```python
from build123d import *

# Parameters (mm, degrees)
F1_DEPTH = 15.24
F2_DEPTH = 12.7
F3_DEPTH = 10.16


with BuildPart() as f1:
    # F0 (on Top) → F1 (new body)
    with BuildSketch(Plane.XY):
        with BuildLine():
            Line((-35.3495, 60.131524), (-40.133959, 60.131524))
            Line((-40.133959, 60.131524), (-40.133959, 43.769562))
            ThreePointArc((-40.133959, 43.769562), (-39.905763, 42.381693), (-39.245203, 41.139955))
            Line((-39.245203, 41.139955), (-26.097199, 34.712043))
            Line((-26.097199, 34.712043), (-26.097199, 60.034128))
            Line((-26.097199, 60.034128), (-30.674654, 60.034128))
            Line((-30.674654, 60.034128), (-30.674654, 42.308667))
            Line((-30.674654, 42.308667), (-30.674654, 42.125131))
            Line((-30.674654, 42.125131), (-34.736989, 43.975933))
            ThreePointArc((-34.736989, 43.975933), (-35.180866, 44.310949), (-35.3495, 44.840879))
            Line((-35.3495, 44.840879), (-35.3495, 60.131524))
        make_face()
        with BuildLine():
            Line((-11.580281, 51.967774), (-6.953094, 49.838448))
            Line((-6.953094, 49.838448), (-6.830248, 58.170216))
            ThreePointArc((-6.830248, 58.170216), (-7.547014, 59.653243), (-9.164316, 59.965426))
            Line((-9.164316, 59.965426), (-19.565252, 59.965426))
            ThreePointArc((-19.565252, 59.965426), (-20.778535, 59.428841), (-21.197871, 58.170216))
            Line((-21.197871, 58.170216), (-21.197871, 47.978059))
            ThreePointArc((-21.197871, 47.978059), (-20.754073, 46.476274), (-19.565252, 45.456952))
            Line((-19.565252, 45.456952), (-11.785025, 41.853478))
            Line((-11.785025, 41.853478), (-11.785025, 35.219812))
            Line((-11.785025, 35.219812), (-14.241938, 34.277995))
            Line((-14.241938, 34.277995), (-16.371263, 35.219812))
            Line((-16.371263, 35.219812), (-16.371263, 39.150875))
            Line((-16.371263, 39.150875), (-21.203195, 41.362097))
            Line((-21.203195, 41.362097), (-21.203195, 34.277995))
            ThreePointArc((-21.203195, 34.277995), (-20.840997, 32.929487), (-19.85189, 31.943927))
            Line((-19.85189, 31.943927), (-13.914351, 29.282272))
            Line((-13.914351, 29.282272), (-8.672934, 31.698236))
            ThreePointArc((-8.672934, 31.698236), (-7.409398, 32.743692), (-6.830248, 34.277995))
            Line((-6.830248, 34.277995), (-6.830248, 43.409521))
            ThreePointArc((-6.830248, 43.409521), (-7.490944, 45.226204), (-9.164316, 46.194026))
            Line((-9.164316, 46.194026), (-16.207468, 49.388015))
            Line((-16.207468, 49.388015), (-16.207468, 55.325555))
            Line((-16.207468, 55.325555), (-11.580281, 55.325555))
            Line((-11.580281, 55.325555), (-11.580281, 51.967774))
        make_face()
        with BuildLine():
            Line((-2.144403, 34.621232), (2.7823, 36.786695))
            Line((2.7823, 36.786695), (2.7823, 41.127243))
            ThreePointArc((2.7823, 41.127243), (3.032611, 41.95286), (3.683167, 42.519495))
            Line((3.683167, 42.519495), (7.368538, 44.239336))
            Line((7.368538, 44.239336), (7.368538, 39.161714))
            Line((7.368538, 39.161714), (10.685371, 40.553966))
            ThreePointArc((10.685371, 40.553966), (11.819683, 41.556771), (12.241417, 43.010876))
            Line((12.241417, 43.010876), (12.241417, 59.792126))
            Line((12.241417, 59.792126), (-0.319427, 59.792126))
            ThreePointArc((-0.319427, 59.792126), (-1.598421, 59.370402), (-2.144403, 58.139313))
            Line((-2.144403, 58.139313), (-2.144403, 34.621232))
        make_face()
        Polygon((2.7823, 47.515221), (2.7823, 55.500185), (7.368538, 55.377342), (7.368538, 49.521698), align=None, mode=Mode.SUBTRACT)
    extrude(amount=F1_DEPTH)


with BuildPart() as f2:
    # F0 (on Top) → F2 (new body)
    with BuildSketch(Plane.XY):
        with BuildLine():
            Line((-36.221196, 34.301637), (-40.116899, 36.103401))
            Line((-40.116899, 36.103401), (-40.26299, 9.51521))
            ThreePointArc((-40.26299, 9.51521), (-38.829457, 4.505833), (-34.924753, 1.055882))
            ThreePointArc((-34.924753, 1.055882), (-35.890099, 3.120786), (-36.221196, 5.376023))
            Line((-36.221196, 5.376023), (-36.221196, 34.301637))
        make_face()
        Polygon((-28.137608, 30.40593), (-32.228097, 32.353785), (-32.053457, -1.11851), (-28.137608, -3.845503), align=None)
        Polygon((-20.025467, 26.800887), (-24.018567, 28.700044), (-24.067261, -6.799573), (-19.834662, -9.769816), align=None)
        Polygon((-14.174307, 24.187266), (-15.983673, 25.047818), (-16.051294, -12.73049), (-13.916418, -14.146952), (-11.990574, -12.73049), (-11.990574, 24.950425), align=None)
        Polygon((-3.661716, 28.700044), (-7.946991, 26.800887), (-7.946991, -9.852093), (-3.476346, -6.828905), align=None)
        Polygon((3.93491, 32.353785), (-0.058187, 30.371067), (-0.058187, -4.008536), (4.109884, -1.182727), align=None)
        with BuildLine():
            Line((12.117932, 36.103401), (7.830616, 33.974593))
            Line((7.830616, 33.974593), (7.984579, 4.465428))
            ThreePointArc((7.984579, 4.465428), (7.646931, 2.635085), (6.661903, 1.055882))
            ThreePointArc((6.661903, 1.055882), (10.736967, 4.274239), (12.258095, 9.23913))
            Line((12.258095, 9.23913), (12.117932, 36.103401))
        make_face()
    extrude(amount=F2_DEPTH)


with BuildPart() as f3:
    # F0 (on Top) → F3 (new body)
    with BuildSketch(Plane.XY):
        with BuildLine():
            Line((17.619875, 65.742654), (-45.880125, 65.742654))
            Line((-45.880125, 65.742654), (-45.880125, 10.423636))
            ThreePointArc((-45.880125, 10.423636), (-44.380848, 3.249228), (-40.133959, -2.724371))
            Line((-40.133959, -2.724371), (-13.956032, -21.107036))
            Line((-13.956032, -21.107036), (13.139814, -1.26348))
            ThreePointArc((13.139814, -1.26348), (16.461486, 4.165449), (17.619875, 10.423636))
            Line((17.619875, 10.423636), (17.619875, 65.742654))
        make_face()
        Polygon((-32.053457, -1.11851), (-32.228097, 32.353785), (-28.137608, 30.40593), (-28.137608, -3.845503), align=None, mode=Mode.SUBTRACT)
        with BuildLine():
            Line((-40.26299, 9.51521), (-40.116899, 36.103401))
            Line((-40.116899, 36.103401), (-36.221196, 34.301637))
            Line((-36.221196, 34.301637), (-36.221196, 5.376023))
            ThreePointArc((-36.221196, 5.376023), (-35.890099, 3.120786), (-34.924753, 1.055882))
            ThreePointArc((-34.924753, 1.055882), (-38.829457, 4.505833), (-40.26299, 9.51521))
        make_face(mode=Mode.SUBTRACT)
        Polygon((-24.067261, -6.799573), (-24.018567, 28.700044), (-20.025467, 26.800887), (-19.834662, -9.769816), align=None, mode=Mode.SUBTRACT)
        Polygon((-16.051294, -12.73049), (-15.983673, 25.047818), (-14.174307, 24.187266), (-11.990574, 24.950425), (-11.990574, -12.73049), (-13.916418, -14.146952), align=None, mode=Mode.SUBTRACT)
        Polygon((-7.946991, -9.852093), (-7.946991, 26.800887), (-3.661716, 28.700044), (-3.476346, -6.828905), align=None, mode=Mode.SUBTRACT)
        Polygon((-0.058187, -4.008536), (-0.058187, 30.371067), (3.93491, 32.353785), (4.109884, -1.182727), align=None, mode=Mode.SUBTRACT)
        with BuildLine():
            Line((7.984579, 4.465428), (7.830616, 33.974593))
            Line((7.830616, 33.974593), (12.117932, 36.103401))
            Line((12.117932, 36.103401), (12.258095, 9.23913))
            ThreePointArc((12.258095, 9.23913), (10.736967, 4.274239), (6.661903, 1.055882))
            ThreePointArc((6.661903, 1.055882), (7.646931, 2.635085), (7.984579, 4.465428))
        make_face(mode=Mode.SUBTRACT)
        with BuildLine():
            Line((-40.133959, 43.769562), (-40.133959, 60.131524))
            Line((-40.133959, 60.131524), (-35.3495, 60.131524))
            Line((-35.3495, 60.131524), (-35.3495, 44.840879))
            ThreePointArc((-35.3495, 44.840879), (-35.180866, 44.310949), (-34.736989, 43.975933))
            Line((-34.736989, 43.975933), (-30.674654, 42.125131))
            Line((-30.674654, 42.125131), (-30.674654, 42.308667))
            Line((-30.674654, 42.308667), (-30.674654, 60.034128))
            Line((-30.674654, 60.034128), (-26.097199, 60.034128))
            Line((-26.097199, 60.034128), (-26.097199, 34.712043))
            Line((-26.097199, 34.712043), (-39.245203, 41.139955))
            ThreePointArc((-39.245203, 41.139955), (-39.905763, 42.381693), (-40.133959, 43.769562))
        make_face(mode=Mode.SUBTRACT)
        with BuildLine():
            Line((-6.830248, 58.170216), (-6.953094, 49.838448))
            Line((-6.953094, 49.838448), (-11.580281, 51.967774))
            Line((-11.580281, 51.967774), (-11.580281, 55.325555))
            Line((-11.580281, 55.325555), (-16.207468, 55.325555))
            Line((-16.207468, 55.325555), (-16.207468, 49.388015))
            Line((-16.207468, 49.388015), (-9.164316, 46.194026))
            ThreePointArc((-9.164316, 46.194026), (-7.490944, 45.226204), (-6.830248, 43.409521))
            Line((-6.830248, 43.409521), (-6.830248, 34.277995))
            ThreePointArc((-6.830248, 34.277995), (-7.409398, 32.743692), (-8.672934, 31.698236))
            Line((-8.672934, 31.698236), (-13.914351, 29.282272))
            Line((-13.914351, 29.282272), (-19.85189, 31.943927))
            ThreePointArc((-19.85189, 31.943927), (-20.840997, 32.929487), (-21.203195, 34.277995))
            Line((-21.203195, 34.277995), (-21.203195, 41.362097))
            Line((-21.203195, 41.362097), (-16.371263, 39.150875))
            Line((-16.371263, 39.150875), (-16.371263, 35.219812))
            Line((-16.371263, 35.219812), (-14.241938, 34.277995))
            Line((-14.241938, 34.277995), (-11.785025, 35.219812))
            Line((-11.785025, 35.219812), (-11.785025, 41.853478))
            Line((-11.785025, 41.853478), (-19.565252, 45.456952))
            ThreePointArc((-19.565252, 45.456952), (-20.754073, 46.476274), (-21.197871, 47.978059))
            Line((-21.197871, 47.978059), (-21.197871, 58.170216))
            ThreePointArc((-21.197871, 58.170216), (-20.778535, 59.428841), (-19.565252, 59.965426))
            Line((-19.565252, 59.965426), (-9.164316, 59.965426))
            ThreePointArc((-9.164316, 59.965426), (-7.547014, 59.653243), (-6.830248, 58.170216))
        make_face(mode=Mode.SUBTRACT)
        with BuildLine():
            Line((2.7823, 41.127243), (2.7823, 36.786695))
            Line((2.7823, 36.786695), (-2.144403, 34.621232))
            Line((-2.144403, 34.621232), (-2.144403, 58.139313))
            ThreePointArc((-2.144403, 58.139313), (-1.598421, 59.370402), (-0.319427, 59.792126))
            Line((-0.319427, 59.792126), (12.241417, 59.792126))
            Line((12.241417, 59.792126), (12.241417, 43.010876))
            ThreePointArc((12.241417, 43.010876), (11.819683, 41.556771), (10.685371, 40.553966))
            Line((10.685371, 40.553966), (7.368538, 39.161714))
            Line((7.368538, 39.161714), (7.368538, 44.239336))
            Line((7.368538, 44.239336), (3.683167, 42.519495))
            ThreePointArc((3.683167, 42.519495), (3.032611, 41.95286), (2.7823, 41.127243))
        make_face(mode=Mode.SUBTRACT)
        Polygon((7.368538, 55.377342), (2.7823, 55.500185), (2.7823, 47.515221), (7.368538, 49.521698), align=None)
    extrude(amount=F3_DEPTH)


with BuildPart() as f2_1:
    add(f2.part)

    # F4: union F3
    add(f3.part)

    # F5: union 


with BuildPart() as f1_1:
    add(f1.part)

    # F6: union F2
    add(f2_1.part)


solid = f1_1.part
```
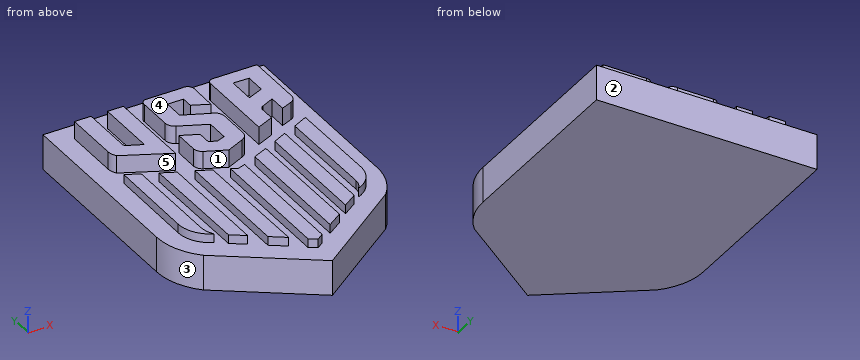
Here's how the part is built. I have some questions about the finished solid (model axes, mm). Face numbers are marked on the shaded views. A direction names the side the tool comes from. Coordinates: 2 decimals unless noted, no trailing zeros. Write each loop counter-clockwise with the first axis right and the second up, starting at its lowest first coordinate (ties: lowest second). Pieces come first, ordered by that corner, then holes. Notation, with made-up numbers: (88.25, 52.5) -> (115.25, 52.5) arc R20 cw to (115.25, 76.5) -> close; hole circle Ø7 at (-38.5, 77). An arc over 180 degrees is marked (long way). Use a Markdown table: item, result. Add a question column.
(1) If we section it at C-C, the plane y = 53: Write out the boundary of the cut face in (x, z), and give its area (3 significant figures).
(2) If we section it at B-B, the plane z = 6: Write out the boundary of the cut face in (x, y), and give its area (3 significant figures).
(3) Please list where these lines run through material, in increasing order: line 1 (X direction, y = -6.5, z = 11.5); line 2 (Z direction, x = 12.5, y = 46.5); line 3 (Y direction, x = 3, z = 10.25).
(4) If we section it at D-D, the plane x = -37.5: Write out the boundary of the cut face in (y, z).
(5) I'm going to push flat-ended pins straight in: P1, Ø2.5, axis at y = 48, z = 12.5, coming from the -X side; P2, Ø3, axis at y = -1.5, z = 11.5, coming from the +X side; P3, Ø5, axis at x = -28, z = 12.5, coming from the +Y side; P4, Ø3.5, axis at x = -6.5, y = 10, coming from the +Z side. Where does each tip first touch, or does it pass through?
(6) We'd pull the mould along Y, two halves only. Please class the marked faces 3, 4 and 5: +Y half, -Y half, draft (parallel to the pull), parting line (faces both ways), or undercut.
(7) If we section it at A-A, the plane z = 14: State how many separate pieces and enclosed holes the cut face has, and give its area (3 significant figures).
(8) For the marked faces 1 and 2, which set-ups out of +Z, -Z, +X, -X, +Y, -Y let a thin tool reach every point of the face, with its end or its side?
Outcome:
| question | item | result |
|---|---|---|
| 1 | outline | (-45.88, 0) -> (17.62, 0) -> (17.62, 10.16) -> (12.24, 10.16) -> (12.24, 15.24) -> (7.37, 15.24) -> (7.37, 10.16) -> (2.78, 10.16) -> (2.78, 15.24) -> (-2.14, 15.24) -> (-2.14, 10.16) -> (-6.91, 10.16) -> (-6.91, 15.24) -> (-11.58, 15.24) -> (-11.58, 10.16) -> (-16.21, 10.16) -> (-16.21, 15.24) -> (-21.2, 15.24) -> (-21.2, 10.16) -> (-26.1, 10.16) -> (-26.1, 15.24) -> (-30.67, 15.24) -> (-30.67, 10.16) -> (-35.35, 10.16) -> (-35.35, 15.24) -> (-40.13, 15.24) -> (-40.13, 10.16) -> (-45.88, 10.16) -> close |
| 1 | area | 792 mm^2 |
| 2 | outline | (-45.88, 10.42) arc R17.92 ccw to (-40.13, -2.72) -> (-13.96, -21.11) -> (13.14, -1.26) arc R17.48 ccw to (17.62, 10.42) -> (17.62, 65.74) -> (-45.88, 65.74) -> close |
| 2 | area | 4,770 mm^2 |
| 3 | line 1 | x = -24.07 to -19.85, -16.04 to -11.99, -7.95 to -3.48 |
| 3 | line 2 | z = 0 to 10.16 |
| 3 | line 3 | y = -1.94 to 31.89, 41.9 to 47.61, 55.49 to 59.79 |
| 4 | outline | (-4.57, 0) -> (65.74, 0) -> (65.74, 10.16) -> (60.13, 10.16) -> (60.13, 15.24) -> (40.29, 15.24) -> (40.29, 10.16) -> (34.89, 10.16) -> (34.89, 12.7) -> (2.85, 12.7) -> (2.85, 10.16) -> (-4.57, 10.16) -> close |
| 5 | P1 | stops at x = -40.13 |
| 5 | P2 | stops at x = 13.52 |
| 5 | P3 | stops at y = 65.74 |
| 5 | P4 | stops at z = 12.7 |
| 6 | face 3 | -Y half |
| 6 | face 4 | draft |
| 6 | face 5 | undercut |
| 7 | separate pieces | 3 |
| 7 | enclosed holes | 1 |
| 7 | area | 785 mm^2 |
| 8 | face 1 | +Z |
| 8 | face 2 | +Z, -Z, +X, -X, +Y |
